Geometry: final body of the model. Coordinates: model frame, mm. A direction names the side the tool comes from. Coordinates: 2 decimals unless noted, no trailing zeros. Loops run counter-clockwise (first coordinate to the right, second up) from the corner with the lowest first, then second, coordinate; pieces in that order, holes last. Notation, with made-up numbers: (71, 81.25) - (109, 81.25) arc R28 ccw to (109, 100.25) - close; hole circle Ø8 at (74.5, -32). An arc over 180 degrees is marked (long way). Answer in a Markdown table with one row per item.
from build123d import *

# Parameters (mm, degrees)
ESQUISSE1_R        = 1.75
BOSS_EXTRU_1_DEPTH = 10
BOSS_EXTRU_2_DEPTH = 2


with BuildPart() as part:
    # Esquisse1 → Boss.-Extru.1 (new body)
    with BuildSketch(Plane.XY):
        Circle(ESQUISSE1_R)
    extrude(amount=BOSS_EXTRU_1_DEPTH)

    # Esquisse2 → Boss.-Extru.2 (add)
    with BuildSketch(Plane.XY.offset(10)):
        Polygon((0, 2.5), (-2.165063509, 1.25), (-2.165063509, -1.25), (0, -2.5), (2.165063509, -1.25), (2.165063509, 1.25), align=None)
    extrude(amount=BOSS_EXTRU_2_DEPTH)


solid = part.part
(1) First-contact query: pin 1 Ø1 at (x, z) = (1.5, 2.5) entering from +Y; pin 2 Ø2 at (y, z) = (-1.5, 7) entering from -X. Flat tips, straight axial feed; report the tip coordinate or a pass-through.
Verdict:
| item | result |
|---|---|
| pin 1 | stops at y = 1.44 |
| pin 2 | stops at x = -1.68 |
(2) Access query for faces 1 (the face through (0, 0, 0)), 2 (the face through (1.617, -0.67, 4.93)). Directions: +Z, -Z, +X, -X, +Y, -Y. A direction counts if a zero-diameter tool reaches every point of the face in a straight line with its end or side. Return the directions, or none.
Verdict:
| item | result |
|---|---|
| face 1 | -Z, +X, -X, +Y, -Y |
| face 2 | -Z |
(3) Cut plane B-B on y = 0. Output: boundary loops of the cut face in (x, z), then the cut area to 3 significant figures.
Verdict:
| item | result |
|---|---|
| outline | (-2.17, 10) - (-1.75, 10) - (-1.75, 0) - (1.75, 0) - (1.75, 10) - (2.17, 10) - (2.17, 12) - (-2.17, 12) - close |
| area | 43.7 mm² |
(4) Cut plane A-A on x = 1.55. Output: boundary loops of the cut face in (y, z), then the cut area to 3 significant figures.
Verdict:
| item | result |
|---|---|
| outline | (-1.61, 10) - (-0.81, 10) - (-0.81, 0) - (0.81, 0) - (0.81, 10) - (1.61, 10) - (1.61, 12) - (-1.61, 12) - close |
| area | 22.7 mm² |
(5) Ray query, probe 1 along Z at (x, y) = (0.7, -1.95); probe 2 along X at (y, z) = (-1.3, 5); probe 3 along X at (y, z) = (-1.45, 1). Return the intervals inside material, ascending.
Verdict:
| item | result |
|---|---|
| probe 1 | z = 10 to 12 |
| probe 2 | x = -1.17 to 1.17 |
| probe 3 | x = -0.98 to 0.98 |
(6) Cut plane C-C on z = 7.25. Output: boundary loops of the cut face in (x, y).
Verdict:
| item | result |
|---|---|
| outline | circle Ø3.5 at (0, 0) |
